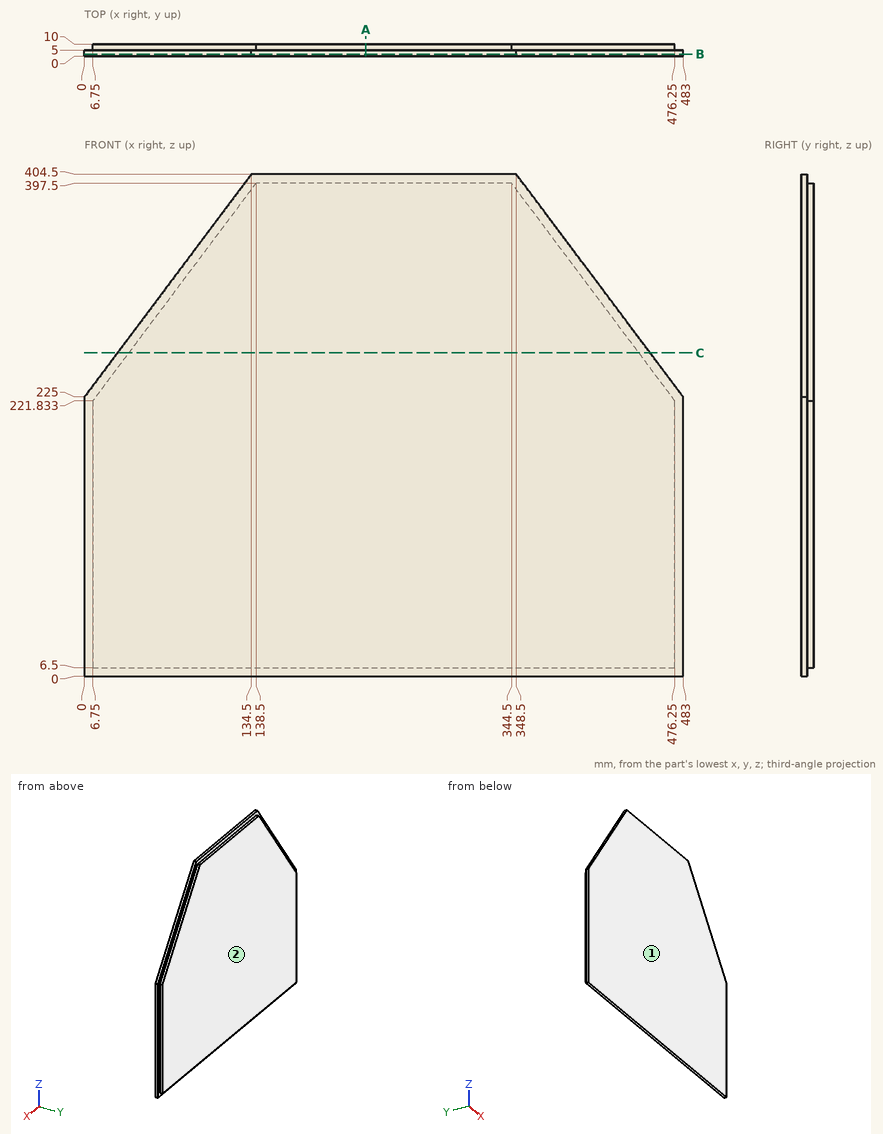
The figure shows three views and two pictorial views of one solid part (mm, origin at its lowest corner). Answer the questions. Give positions to 0.01 mm unless a question says otherwise; leave off trailing zeros. Order: outer loops, then holes, each group sorted by start corner. A loop starts at its lowest first (then second) coordinate and runs counter-clockwise, first axis right, second up. Notation, with made-up numbers: M 84,19 L 135,19 A19 ccw 135,55 Z; hole C 79.5,18 d5. An arc over 180 degrees is marked long. Return JSON: item names as keys, results as strings.
Q1. Find section B-B, the plane y = 1.75. Write down the section's boundary in (x, z), and give its area (3 significant figures).
Answer below:
{"outline": "M 0,0 L 483,0 L 483,225 L 348.5,404.5 L 134.5,404.5 L 0,225 Z", "area": "171,000 mm^2"}
Q2. The mould has two halves that part along Y. Classify the marked faces 1 and 2: pulls with the +Y half, pulls with the -Y half, needs draft (parallel to the pull), parting line crosses it, or undercut.
Answer below:
{"face 1": "pulls with the -Y half", "face 2": "pulls with the +Y half"}
Q3. Find section A-A, the plane x = 227. Write down the section's boundary in (y, z), and give its area (3 significant figures).
Answer below:
{"outline": "M 0,0 L 5,0 L 5,6.5 L 10,6.5 L 10,397.5 L 5,397.5 L 5,404.5 L 0,404.5 Z", "area": "3,980 mm^2"}
Q4. Each of these flat-tipped pins is pushed along its axis until it touches: pin 1 (2.5 mm diameter, centred on x = 340, y = 8, fed in from -Z); pin 2 (3 mm diameter, centred on y = 8, z = 239.5, fed in from +X) (1 decimal); pin 3 (6 mm diameter, centred on y = 2, z = 286.5, fed in from -X) (1 decimal); pin 4 (5 mm diameter, centred on y = 6.5, z = 172.5, fed in from +X). Where does it stop, or does it pass through?
Answer below:
{"pin 1": "stops at z = 6.5", "pin 2": "stops at x = 464.1", "pin 3": "stops at x = 43.8", "pin 4": "stops at x = 483"}
Q5. Find the intervals of material crossed by line 1 along X through (y, z) = (5.25, 207); line 2 along Z through (x, y) = (245.5, 5.25); line 3 along Z through (x, y) = (75.5, 1), in increasing order. Write a range as [from, to].
Answer below:
{"line 1": "x = [6.75, 476.25]", "line 2": "z = [6.5, 397.5]", "line 3": "z = [0, 325.76]"}
Q6. Find section C-C, the plane z = 260.5. Write down the section's boundary in (x, y), and give its area (3 significant figures).
Answer below:
{"outline": "M 26.6,0 L 456.4,0 L 456.4,5 L 447.25,5 L 447.25,10 L 35.75,10 L 35.75,5 L 26.6,5 Z", "area": "4,210 mm^2"}
